Source: CAD feature listing. Evaluate the final solid. Frame: model axes, mm. A direction names the side the tool comes from. Give positions to 0.01 mm unless a question says otherwise; leave off trailing zeros. Order: outer loops, then holes, each group sorted by start corner. A loop starts at its lowest first (then second) coordinate and runs counter-clockwise, first axis right, second up. Notation, with made-up numbers: M -11.5,33 L 26.5,33 A28 ccw 26.5,64 Z; hole C 46,-8 d8. An arc over 180 degrees is marked long. Use CSV: the item, a comma, the result in double quotes. Start each with the question number.
1. Reachability of faces 4 (the flat face through (53, 65, 2)), 5 (the flat face through (15, 62, 2)), 6 (the flat face through (7, 0, 2)) from +Z, -Z, +X, -X, +Y, -Y: full face, straight path, thin tool, end or side. Return the list, or none.
2. Line query: line 1 along X through (y, z) = (-6, 1.1); line 2 along Y through (x, z) = (27.5, 3.55); line 3 along Y through (x, z) = (13.5, 1.7). Output: solid intervals per line, ascending. Write a range as [from, to].
3. Pin query (flat end, axial travel): P1, Ø1.5, axis at x = 18, z = 3.5, coming from the -Y side; P2, Ø2, axis at x = 38.5, z = 2.5, coming from the +Y side. Return the tip coordinate at first contact, or that it passes through.
4. Section query B-B, the plane x = 13.5. Return the cut outline in (y, z), plus the area to 4 significant figures.
5. Mould query, pull axis X, two halves, no side actions, for faces 1 (the flat face through (3, 65, 2)), 2 (the flat face through (50, -5, 2)), 3 (the flat face through (27, 0, 2)). Classes: released by +X, released by -X, zero draft, split by the parting line, or undercut.
6. Section query D-D, the plane x = 47.5. Return the cut outline in (y, z).
7. Section query C-C, the plane z = 3.05. State how many separate pieces and enclosed holes the cut face has, plus the area to 3 significant figures.
8. Section query A-A, the plane y = 37. Return the cut outline in (x, z).
from build123d import *

# Parameters (mm, degrees)
ESQUISSE1_R        = 1.25
ESQUISSE1_R_2      = 6
BOSS_EXTRU_1_DEPTH = 5


with BuildPart() as part:
    # Esquisse1 → Boss.-Extru.1 (new body)
    with BuildSketch(Plane.XY):
        Polygon((15, 65), (10, 65), (10, 60), (5, 60), (5, 65), (0, 65), (0, -10), (5, -10), (5, 0), (10, 0), (10, -10), (15, -10), (15, 0), (20, 0), (20, -10), (25, -10), (25, 0), (30, 0), (30, -10), (35, -10), (35, 0), (40, 0), (40, -10), (45, -10), (45, 0), (50, 0), (50, -10), (55, -10), (55, 65), (50, 65), (50, 60), (45, 60), (45, 65), (40, 65), (40, 60), (35, 60), (35, 65), (30, 65), (30, 60), (25, 60), (25, 65), (20, 65), (20, 60), (15, 60), align=None)
        with Locations((41.5, 30)):
            Circle(ESQUISSE1_R, mode=Mode.SUBTRACT)
        with Locations((13.5, 30)):
            Circle(ESQUISSE1_R, mode=Mode.SUBTRACT)
        with Locations((27.5, 37)):
            Circle(ESQUISSE1_R_2, mode=Mode.SUBTRACT)
    extrude(amount=BOSS_EXTRU_1_DEPTH)


solid = part.part
Result set:
1,face 4,"+Z, -Z, +X, -X, +Y"
1,face 5,"+Z, -Z, +Y"
1,face 6,"+Z, -Z, -Y"
2,line 1,"[0, 5], [10, 15], [20, 25], [30, 35], [40, 45], [50, 55]"
2,line 2,"[0, 31], [43, 60]"
2,line 3,"[-10, 28.75], [31.25, 65]"
3,P1,"y = 0"
3,P2,"y = 60"
4,outline,"M -10,0 L 28.75,0 L 28.75,5 L -10,5 Z; M 31.25,0 L 65,0 L 65,5 L 31.25,5 Z"
4,area,"362.5 mm2"
5,face 1,"zero draft"
5,face 2,"undercut"
5,face 3,"undercut"
6,outline,"M 0,0 L 60,0 L 60,5 L 0,5 Z"
7,separate pieces,"1"
7,enclosed holes,"3"
7,area,"3,630 mm2"
8,outline,"M 0,0 L 21.5,0 L 21.5,5 L 0,5 Z; M 33.5,0 L 55,0 L 55,5 L 33.5,5 Z"
